For this review, take the finished solid that the model builds, in its own axes (mm). Face numbers are marked on the shaded views. A direction names the side the tool comes from. Round coordinates to 2 decimals unless told otherwise and drop trailing zeros. Write each loop counter-clockwise with the first axis right and the second up, starting at its lowest first coordinate (ties: lowest second). Pieces come first, ordered by that corner, then holes. Notation, with made-up numbers: (25.25, 8.25) -> (52.25, 8.25) arc R8 ccw to (52.25, 22.25) -> close; hole circle Ø8 at (66.5, -30.75). An arc over 180 degrees is marked (long way). Answer in a Markdown table with one row per item.
from build123d import *

# Parameters (mm, degrees)
CROQUIS2_R              = 18
SALIENTE_EXTRUIR1_DEPTH = 30
CROQUIS3_R              = 13
SALIENTE_EXTRUIR3_DEPTH = 10
CROQUIS5_R              = 8
SALIENTE_EXTRUIR4_DEPTH = 20
CROQUIS6_OUTSIDE_W      = 69.738
CROQUIS6_OUTSIDE_H      = 69.738
CROQUIS6_OUTSIDE_R      = 13
CORTAR_EXTRUIR2_DEPTH   = 8
CORTAR_EXTRUIR2_DRAFT   = -45
CROQUIS7_OUTSIDE_W      = 76.588
CROQUIS7_OUTSIDE_H      = 76.588
CROQUIS7_OUTSIDE_R      = 8
CORTAR_EXTRUIR5_DEPTH   = 8
CORTAR_EXTRUIR5_DRAFT   = -55
CROQUIS8_R              = 19
SALIENTE_EXTRUIR5_DEPTH = 3
CROQUIS9_R              = 1.5
CORTAR_EXTRUIR6_DEPTH   = 3


with BuildPart() as part:
    # Croquis2 → Saliente-Extruir1 (new body)
    with BuildSketch(Plane.XY):
        Circle(CROQUIS2_R)
    extrude(amount=SALIENTE_EXTRUIR1_DEPTH)

    # Croquis3 → Saliente-Extruir3 (add)
    with BuildSketch(Plane.XY.offset(30)):
        Circle(CROQUIS3_R)
    extrude(amount=SALIENTE_EXTRUIR3_DEPTH)

    # Croquis5 → Saliente-Extruir4 (add)
    with BuildSketch(Plane(origin=(0, 0, 0), x_dir=(-1, 0, 0), z_dir=(0, 0, -1))):
        Circle(CROQUIS5_R)
    extrude(amount=SALIENTE_EXTRUIR4_DEPTH)


with BuildPart() as cortar_extruir2_tool:
    # Croquis6 outside → Cortar-Extruir2 (with draft: the straight prism first)
    with BuildSketch(Plane.XY.offset(30)):
        Rectangle(CROQUIS6_OUTSIDE_W, CROQUIS6_OUTSIDE_H)
        Circle(CROQUIS6_OUTSIDE_R, mode=Mode.SUBTRACT)
    extrude(amount=-CORTAR_EXTRUIR2_DEPTH)
    # Cortar-Extruir2: the draft: its side faces are tilted about the plane it starts from
    cortar_extruir2_sides = [cortar_extruir2_tool.faces().sort_by_distance(p)[0] for p in [
        (0, -34.869, 26),
        (34.869, 0, 26),
        (0, 34.869, 26),
        (-34.869, 0, 26),
        (-13, 0, 26),
    ]]
    draft(cortar_extruir2_sides, Plane.XY.offset(30), CORTAR_EXTRUIR2_DRAFT)


with BuildPart() as part_1:
    add(part.part)

    # Cortar-Extruir2: cut by cortar_extruir2_tool
    add(cortar_extruir2_tool.part, mode=Mode.SUBTRACT)


with BuildPart() as cortar_extruir5_tool:
    # Croquis7 outside → Cortar-Extruir5 (with draft: the straight prism first)
    with BuildSketch(Plane(origin=(0, 0, 0), x_dir=(-1, 0, 0), z_dir=(0, 0, -1))):
        Rectangle(CROQUIS7_OUTSIDE_W, CROQUIS7_OUTSIDE_H)
        Circle(CROQUIS7_OUTSIDE_R, mode=Mode.SUBTRACT)
    extrude(amount=-CORTAR_EXTRUIR5_DEPTH)
    # Cortar-Extruir5: the draft: its side faces are tilted about the plane it starts from
    cortar_extruir5_sides = [cortar_extruir5_tool.faces().sort_by_distance(p)[0] for p in [
        (0, -38.294, 4),
        (-38.294, 0, 4),
        (0, 38.294, 4),
        (38.294, 0, 4),
        (8, 0, 4),
    ]]
    draft(cortar_extruir5_sides, Plane(origin=(0, 0, 0), x_dir=(-1, 0, 0), z_dir=(0, 0, -1)), CORTAR_EXTRUIR5_DRAFT)


with BuildPart() as part_2:
    add(part_1.part)

    # Cortar-Extruir5: cut by cortar_extruir5_tool
    add(cortar_extruir5_tool.part, mode=Mode.SUBTRACT)

    # Croquis8 → Saliente-Extruir5 (add)
    with BuildSketch(Plane.XY.offset(40)):
        Circle(CROQUIS8_R)
    extrude(amount=SALIENTE_EXTRUIR5_DEPTH)

    # Croquis9 → Cortar-Extruir6 (cut)
    with BuildSketch(Plane.XY.offset(43)):
        with Locations((0, 16)):
            Circle(CROQUIS9_R)
        with Locations((13.856406461, 8)):
            Circle(CROQUIS9_R)
        with Locations((13.856406461, -8)):
            Circle(CROQUIS9_R)
        with Locations((0, -16)):
            Circle(CROQUIS9_R)
        with Locations((-13.856406461, -8)):
            Circle(CROQUIS9_R)
        with Locations((-13.856406461, 8)):
            Circle(CROQUIS9_R)
    extrude(amount=-CORTAR_EXTRUIR6_DEPTH, mode=Mode.SUBTRACT)


solid = part_2.part
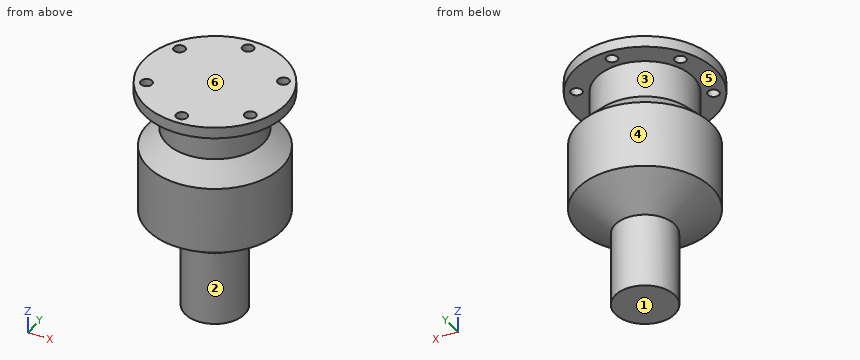
1) Consider section C-C on y = -16. State how many separate pieces and enclosed holes the cut face has, then the cut area to 3 significant figures.
Solved:
| item | result |
|---|---|
| separate pieces | 3 |
| enclosed holes | 0 |
| area | 386 mm² |
2) Consider section B-B on z = -1. State the section outline as (x, y) points, then the cut area to 3 significant figures.
Solved:
| item | result |
|---|---|
| outline | circle Ø16 at (0, 0) |
| area | 201 mm² |
3) Clearance check with flat-ended pins moving along their axes: pin 1 Ø5 at (x, y) = (0, -16) entering from -Z; pin 2 Ø2.5 at (x, y) = (13.86, 8) entering from -Z; pin 3 Ø10 at (y, z) = (7.5, -10.5) entering from +X. State where each tip first meets the part, or that it passes through.
Solved:
| item | result |
|---|---|
| pin 1 | z = 3.85 |
| pin 2 | z = 4.73 |
| pin 3 | x = 7.6 |
4) Mouldability with a two-part tool opening along Z and no side actions: class the marked faces 4, 5 and 6 as pulls with the +Z half, pulls with the -Z half, needs draft (parallel to the pull), parting line crosses it, or undercut.
Solved:
| item | result |
|---|---|
| face 4 | needs draft |
| face 5 | undercut |
| face 6 | pulls with the +Z half |
5) For line 1 (Y direction, x = 0, z = 41.95); line 2 (Z direction, x = -14.5, y = -10.5); line 3 (Z direction, x = 15.5, y = -7), list the stretches that pass through material, from the lowest coordinate up. Write a range as [from, to].
Solved:
| item | result |
|---|---|
| line 1 | [-19, -17.5], [-14.5, 14.5], [17.5, 19] |
| line 2 | [6.93, 25.1], [40, 43] |
| line 3 | [6.31, 25.99], [40, 43] |
6) Consider section D-D on z = 14.5. State the section outline as (x, y) points, then the cut area to 3 significant figures.
Solved:
| item | result |
|---|---|
| outline | circle Ø36 at (0, 0) |
| area | 1,020 mm² |
7) For the marked faces 1, 2 and 3, list the 3-axis set-ups (+Z, -Z, +X, -X, +Y, -Y) from which the entire face can be reached by the end or side of a thin tool; tool diameter is ignored.
Solved:
| item | result |
|---|---|
| face 1 | -Z, +X, -X, +Y, -Y |
| face 2 | -Z |
| face 3 | none |
8) Consider section A-A on x = 0. State the section outline as (y, z) points.
Solved:
| item | result |
|---|---|
| outline | (-19, 40) -> (-17.5, 40) -> (-17.5, 43) -> (-19, 43) -> close; (-18, 7) -> (-8, 0) -> (-8, -20) -> (8, -20) -> (8, 0) -> (18, 7) -> (18, 25) -> (13, 30) -> (13, 40) -> (14.5, 40) -> (14.5, 43) -> (-14.5, 43) -> (-14.5, 40) -> (-13, 40) -> (-13, 30) -> (-18, 25) -> close; (17.5, 40) -> (19, 40) -> (19, 43) -> (17.5, 43) -> close |
